Input: part model. Units: mm. Frame: model coordinates. A direction names the side the tool comes from. Coordinates: 2 decimals unless noted, no trailing zeros. Use a Markdown table: item, result. Add a question column.
1. Line query: L1, parallel to Z at x = -0.15, y = 16; L2, parallel to X at y = 37.5, z = 0; L3, parallel to Z at x = -0.65, y = 23. Output: solid intervals per line, ascending. Write a range as [from, to].
2. Set-up query: faces 3 (the conical face through (-0.37, 5.68, -1.16)), 4 (the conical face through (2.342, 20.754, 0.52)). Return all of +Z, -Z, +X, -X, +Y, -Y with unobstructed straight access to the full face (end or side cutting, diameter ignored); none if empty.
3. Draft query along Z for faces 1 (the conical face through (-0.782, 20.796, -2.484)), 2 (the cylindrical face through (-0.811, 52.599, -2.575)). Return one class per face: +Z half, -Z half, draft (parallel to the pull), parting line (faces both ways), or undercut.
4. Pin query (flat end, axial travel): pin 1 (1.5 mm diameter, centred on x = 1.5, y = 33, fed in from +Z); pin 2 (1.5 mm diameter, centred on x = -2, y = 20.5, fed in from -Z); pin 3 (1 mm diameter, centred on x = 0.5, y = 58, fed in from -Z); pin 4 (2 mm diameter, centred on x = -1.5, y = 27.5, fed in from +Z). Return the tip coordinate at first contact, or that it passes through.
```python
from build123d import *


with BuildPart() as part:
    # Sketch1 → Base-Revolve (revolve)
    with BuildSketch(Plane.XY, mode=Mode.PRIVATE) as base_revolve_sk:
        Polygon((-0.99999907, 0), (-1.2, 0), (-1.25, 16.399999998), (-2.3, 17.5), (-2.9, 24), (-2.9, 82), (-2.7, 82), (-2.7, 24.00921119), (-2.107247336, 17.587723996), (-1.050244154, 16.480387327), align=None)
    revolve(base_revolve_sk.sketch.rotate(Axis((0, 0, 0), (0, 1, 0)), 270), axis=Axis((0, 0, 0), (0, 1, 0)))

    # Esboço1 → Revolução1 (revolve)
    with BuildSketch(Plane.XY, mode=Mode.PRIVATE) as revolu_o1_sk:
        Polygon((-1.234146341, 11.2), (-1.3, 11.314061882), (-1.3, 16.45238095), (-1.25, 16.399999998), align=None)
    revolve(revolu_o1_sk.sketch.rotate(Axis((0, 0, 0), (0, 1, 0)), 90), axis=Axis((0, 0, 0), (0, 1, 0)))


solid = part.part
```
Answers below:
| question | item | result |
|---|---|---|
| 1 | L1 | z = [-1.29, -1.04], [1.04, 1.29] |
| 1 | L2 | x = [-2.9, -2.7], [2.7, 2.9] |
| 1 | L3 | z = [-2.73, -2.52], [2.52, 2.73] |
| 2 | face 3 | -Y |
| 2 | face 4 | +Y |
| 3 | face 1 | parting line |
| 3 | face 2 | undercut |
| 4 | pin 1 | stops at z = 2.8 |
| 4 | pin 2 | stops at z = -2.26 |
| 4 | pin 3 | stops at z = -2.9 |
| 4 | pin 4 | stops at z = 2.86 |
